```python
from build123d import *

# Parameters (mm, degrees)
CROQUIS1_R              = 10
SALIENTE_EXTRUIR1_DEPTH = 250
CROQUIS3_W              = 200
CROQUIS3_H              = 161.5
CORTAR_EXTRUIR1_DEPTH   = 250


with BuildPart() as part:
    # Croquis1 → Saliente-Extruir1 (new body)
    with BuildSketch(Plane.XY):
        with BuildLine():
            Line((0, 150), (0, 250))
            ThreePointArc((0, 250), (24.449494329, 286.853517788), (67.909088668, 278.654541869))
            Line((67.909088668, 278.654541869), (200, 150))
            Line((200, 150), (200, 0))
            Line((200, 0), (0, 0))
            Line((0, 0), (0, 150))
        make_face()
        with Locations((40, 250)):
            Circle(CROQUIS1_R, mode=Mode.SUBTRACT)
    extrude(amount=SALIENTE_EXTRUIR1_DEPTH)

    # Croquis3 → Cortar-Extruir1 (cut)
    with BuildSketch(Plane.ZY):
        with Locations((125, 209.25)):
            Rectangle(CROQUIS3_W, CROQUIS3_H)
    extrude(amount=-CORTAR_EXTRUIR1_DEPTH, mode=Mode.SUBTRACT)


solid = part.part
```
Design review of the part built by this model. Coordinates are the model's own, in mm. A direction names the side the tool comes from. Round coordinates to 2 decimals unless told otherwise and drop trailing zeros. Write each loop counter-clockwise with the first axis right and the second up, starting at its lowest first coordinate (ties: lowest second). Pieces come first, ordered by that corner, then holes. Notation, with made-up numbers: (26, 42) -> (35, 42) arc R21 cw to (35, 47) -> close; hole circle Ø5 at (-5.5, -1). An arc over 180 degrees is marked (long way). Answer in a Markdown table with one row per item.
Q1. Take a section at D-D, the plane z = 191.5. State the section outline as (x, y) points, then the cut area to 3 significant figures.
The answers:
| item | result |
|---|---|
| outline | (0, 0) -> (200, 0) -> (200, 128.5) -> (0, 128.5) -> close |
| area | 25,700 mm² |
Q2. Take a section at C-C, the plane x = 152.5. State the section outline as (y, z) points, then the cut area to 3 significant figures.
The answers:
| item | result |
|---|---|
| outline | (0, 0) -> (196.26, 0) -> (196.26, 25) -> (128.5, 25) -> (128.5, 225) -> (196.26, 225) -> (196.26, 250) -> (0, 250) -> close |
| area | 35,500 mm² |
Q3. Draft analysis for pull direction Y (two halves, no side actions). For faces 1 (the face through (38.698, 259.915, 12.325)), 2 (the face through (133.03, 215.23, 12.32)), 3 (the face through (38.698, 259.915, 237.325)), 4 (the face through (76, 190, 225)), state which applies: +Y half, -Y half, draft (parallel to the pull), parting line (faces both ways), or undercut.
The answers:
| item | result |
|---|---|
| face 1 | undercut |
| face 2 | +Y half |
| face 3 | undercut |
| face 4 | draft |
Q4. Take a section at A-A, the plane x = 40. State the section outline as (y, z) points.
The answers:
| item | result |
|---|---|
| outline | (0, 0) -> (240, 0) -> (240, 25) -> (128.5, 25) -> (128.5, 225) -> (240, 225) -> (240, 250) -> (0, 250) -> close; (260, 0) -> (290, 0) -> (290, 25) -> (260, 25) -> close; (260, 225) -> (290, 225) -> (290, 250) -> (260, 250) -> close |
Q5. To check wall thickness, follow L1, parallel to Z at x = 81, y = 198.5; L2, parallel to Y at x = 40, z = 231; L3, parallel to Y at x = 21, z = 132.5. State the ranges of each line that lie inside material, in increasing order. Write a range as [from, to].
The answers:
| item | result |
|---|---|
| L1 | [0, 25], [225, 250] |
| L2 | [0, 240], [260, 290] |
| L3 | [0, 128.5] |
Q6. Take a section at B-B, the plane y = 265. State the section outline as (x, z) points.
The answers:
| item | result |
|---|---|
| outline | (2.92, 0) -> (81.93, 0) -> (81.93, 25) -> (2.92, 25) -> close; (2.92, 225) -> (81.93, 225) -> (81.93, 250) -> (2.92, 250) -> close |
Q7. For faces 5 (the face through (101, 115, 250)), 6 (the face through (99, 128.5, 124)), list the 3-axis set-ups (+Z, -Z, +X, -X, +Y, -Y) from which the entire face can be reached by the end or side of a thin tool; tool diameter is ignored.
The answers:
| item | result |
|---|---|
| face 5 | +Z, +X, -X, +Y, -Y |
| face 6 | +X, -X, +Y |
Q8. Clearance check with a flat-ended pin moving along its axis: pin 1 Ø2 at (x, z) = (41, 172) entering from +Y. State where the tip first meets the part, or that it passes through.
The answers:
| item | result |
|---|---|
| pin 1 | y = 128.5 |
